Input: dimensioned drawing with shaded views. Units: mm. Origin: part minimum x, y, z. A direction names the side the tool comes from. Coordinates: 2 decimals unless noted, no trailing zeros. Order: outer loops, then holes, each group sorted by start corner. A loop starts at its lowest first (then second) coordinate and runs counter-clockwise, first axis right, second up. Notation, with made-up numbers: (34.5, 21) - (38.5, 21) arc R10 ccw to (38.5, 29) - close; hole circle Ø5 at (-32.75, 18.5). An arc over 180 degrees is marked (long way). One line per question, with ' | ' between items. Start each with the question number.
(1) Section D-D (z = 1.75). Return the cut outline in (x, y).
(2) Section A-A (x = 7). Return the cut outline in (y, z), then the cut area to 3 significant figures.
(3) Access query for the marked faces 4 and 5. Directions: +Z, -Z, +X, -X, +Y, -Y. A direction counts if a zero-diameter tool reaches every point of the face in a straight line with its end or side. Return the directions, or none.
(4) Draft query along X for the marked faces 1, 2 and 3. Return one class per face: +X half, -X half, draft (parallel to the pull), parting line (faces both ways), or undercut.
(5) Line query: line 1 along Y through (x, z) = (7, 11.1); line 2 along Y through (x, z) = (13, 6); line 3 along X through (y, z) = (3.75, 7.75). Output: solid intervals per line, ascending.
(6) Section C-C (y = 3). Return the cut outline in (x, z).
(7) Contact query for a flat-ended pin moving along its axis: P1, Ø2, axis at y = 3.5, z = 8, coming from the -X side. Output: stop coordinate, or through.
(8) Section B-B (z = 7). Return the cut outline in (x, y), then the cut area to 3 significant figures.
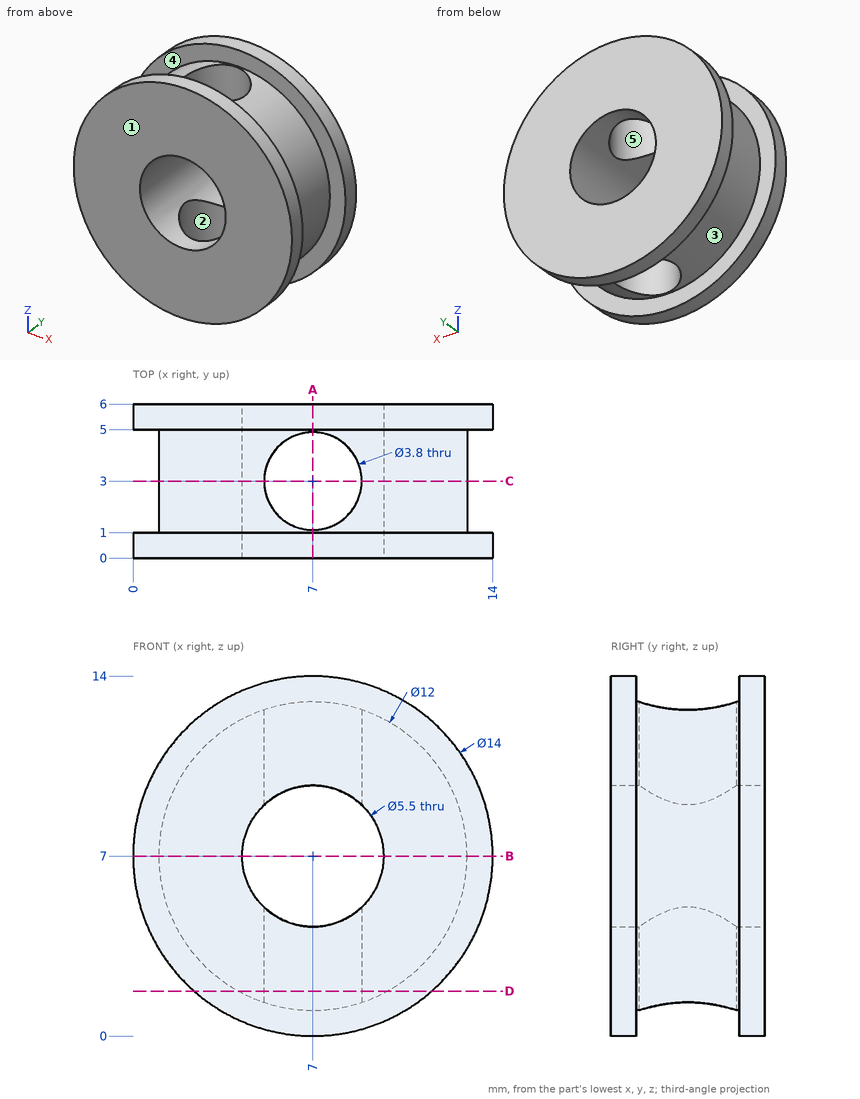
Response values:
1) outline: (2.37, 0) - (11.63, 0) - (11.63, 1) - (9.9, 1) - (9.9, 5) - (11.63, 5) - (11.63, 6) - (2.37, 6) - (2.37, 5) - (4.1, 5) - (4.1, 1) - (2.37, 1) - close; hole circle Ø3.8 at (7, 3)
2) outline: (0, 0) - (1, 0) - (1, 1) - (1.1, 1) - (1.1, 4.25) - (0, 4.25) - close; (0, 9.75) - (1.1, 9.75) - (1.1, 13) - (1, 13) - (1, 14) - (0, 14) - close; (4.9, 1) - (5, 1) - (5, 0) - (6, 0) - (6, 4.25) - (4.9, 4.25) - close; (4.9, 9.75) - (6, 9.75) - (6, 14) - (5, 14) - (5, 13) - (4.9, 13) - close | area: 18.3 mm²
3) face 4: none | face 5: +Z, -Z
4) face 1: draft | face 2: undercut | face 3: parting line
5) line 1: y = 0 to 1.1, 4.9 to 6 | line 2: y = 0 to 1, 5 to 6 | line 3: x = 1.05 to 4.35, 9.65 to 12.95
6) outline: (5.1, 1.31) - (5.1, 5.01) arc R2.75 cw to (5.1, 8.99) - (5.1, 12.69) arc R6 ccw to start; (8.9, 1.31) arc R6 ccw to (8.9, 12.69) - (8.9, 8.99) arc R2.75 cw to (8.9, 5.01) - close
7) P1: stops at x = 1
8) outline: (0, 0) - (4.25, 0) - (4.25, 6) - (0, 6) - (0, 5) - (1, 5) - (1, 1) - (0, 1) - close; (9.75, 0) - (14, 0) - (14, 1) - (13, 1) - (13, 5) - (14, 5) - (14, 6) - (9.75, 6) - close | area: 43.0 mm²
